Could you check a few things on this model? Use its own coordinates, in mm. Give positions to 0.01 mm unless a question says otherwise; leave off trailing zeros. Write each loop counter-clockwise with the first axis right and the second up, starting at its lowest first coordinate (ties: lowest second). Pieces come first, ordered by that corner, then holes. Notation, with made-up numbers: M -8.75,35 L 50.25,35 A30 ccw 50.25,72 Z; hole C 7.25,32.25 d6. An arc over 180 degrees is marked long. One line per item, written item: value.
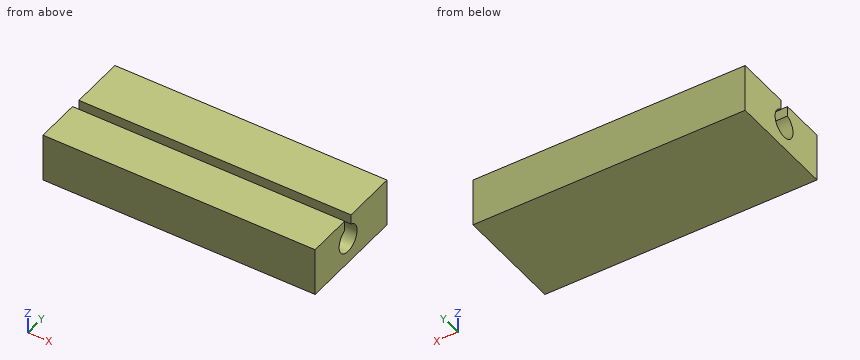
```python
from build123d import *

# Parameters (mm, degrees)
F0_W     = 126.748518
F0_H     = 22.633665
F1_DEPTH = 50.8
F3_D     = 12.7
F4_W     = 4.541321
F4_H     = 4.775913
F5_DEPTH = 254


with BuildPart() as f1:
    # F0 (on Front) → F1 (new body)
    with BuildSketch(Plane.XZ):
        with Locations((7.582277, -0.67901)):
            Rectangle(F0_W, F0_H)
    extrude(amount=F1_DEPTH)

    # F3 (through all)
    with Locations(Plane(origin=(-55.791982, 0, 0), x_dir=(0, -1, 0), z_dir=(-1, 0, 0))):
        with Locations((27.499903, 0)):
            Hole(F3_D / 2)

    # F4 (on face) → F5 (cut)
    with BuildSketch(Plane(origin=(-55.791982, 0, 0), x_dir=(0, -1, 0), z_dir=(-1, 0, 0))):
        with Locations((27.67066, 8.249866)):
            Rectangle(F4_W, F4_H)
    extrude(amount=-F5_DEPTH, mode=Mode.SUBTRACT)


solid = f1.part
```
1) If we section it at A-A, the plane z = 0: Write out the boundary of the cut face in (x, y).
Outcome:
outline: M -55.79,-50.8 L 70.96,-50.8 L 70.96,-33.85 L -55.79,-33.85 Z; M -55.79,-21.15 L 70.96,-21.15 L 70.96,0 L -55.79,0 Z
2) If we section it at C-C, the plane x = 9: Write out the boundary of the cut face in (y, z), then the cut area to 3 significant figures.
Outcome:
outline: M -50.8,-12 L 0,-12 L 0,10.64 L -25.4,10.64 L -25.4,5.99 A6.35 cw long -29.94,5.86 L -29.94,10.64 L -50.8,10.64 Z
area: 1,000 mm^2
3) Please list where these lines run through material, in increasing order: L1, parallel to Y at x = 32.5, z = 9.25; L2, parallel to Y at x = -15, z = 0; L3, parallel to Z at x = 62, y = -29. Write a range as from..to.
Outcome:
L1: y = -50.8..-29.94, -25.4..0
L2: y = -50.8..-33.85, -21.15..0
L3: z = -12..-6.17
4) If we section it at B-B, the plane y = -32.5: Write out the boundary of the cut face in (x, z), then the cut area to 3 significant figures.
Outcome:
outline: M -55.79,-12 L 70.96,-12 L 70.96,-3.91 L -55.79,-3.91 Z; M -55.79,3.91 L 70.96,3.91 L 70.96,10.64 L -55.79,10.64 Z
area: 1,880 mm^2
5) I'm going to push a flat-ended pin straight in: pin 1 (5 mm diameter, centred on x = -6, z = -8.5, fed in from +Y). Where does the tip first touch, or does it pass through?
Outcome:
pin 1: stops at y = 0
